Check sheet for the drawn part. Datum: minimum x, y, z corner. Units: mm. A direction names the side the tool comes from. Give positions to 0.01 mm unless a question says otherwise; leave off trailing zeros. Write each loop counter-clockwise with the first axis right and the second up, starting at its lowest first coordinate (ties: lowest second). Pieces come first, ordered by that corner, then holes. Notation, with made-up numbers: M -10,12 L -6,12 A25 ccw -6,38 Z; hole C -14,-28 d2. An arc over 180 degrees is marked long. Write item = value, one per line.
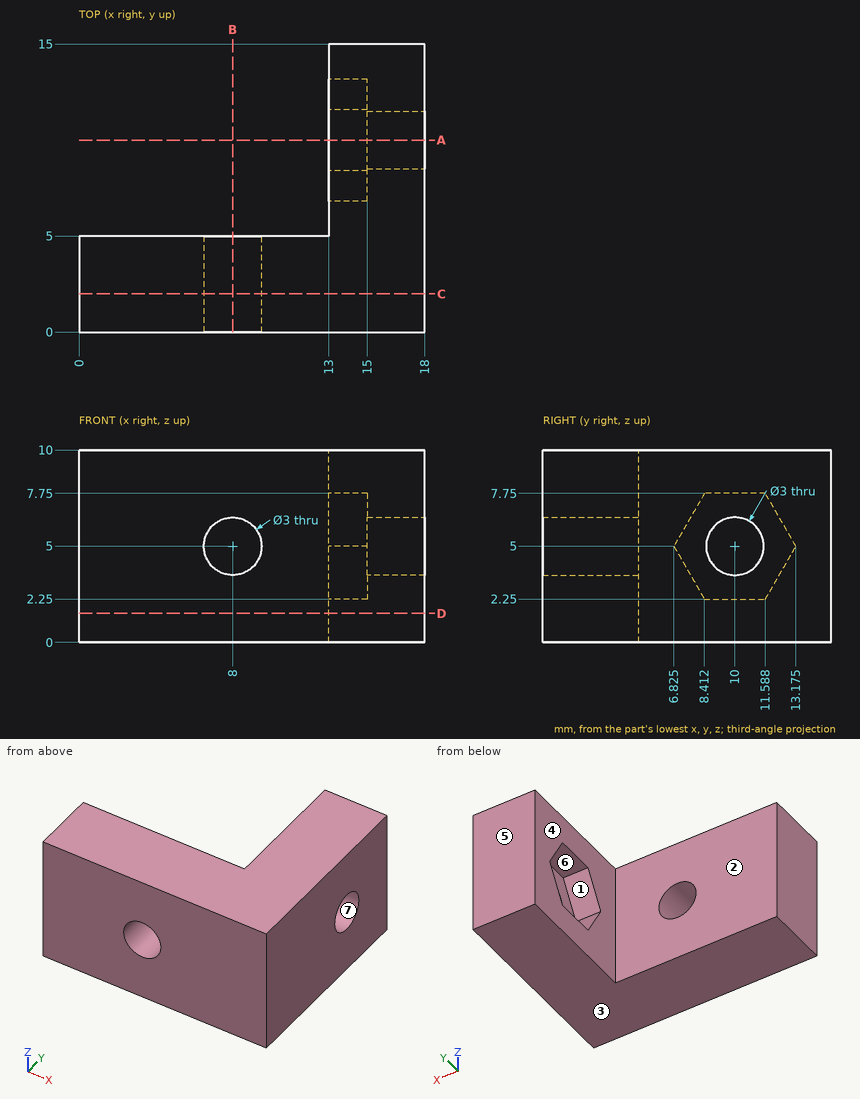
1) Cross-section at C-C on y = 2. Record the boundary of the cut face in (x, z).
From the geometry:
outline = M 0,0 L 18,0 L 18,10 L 0,10 Z; hole C 8,5 d3
2) Cross-section at A-A on y = 10. Record the boundary of the cut face in (x, z), plus the area to 3 significant figures.
From the geometry:
outline = M 13,0 L 18,0 L 18,3.5 L 15,3.5 L 15,2.25 L 13,2.25 Z; M 13,7.75 L 15,7.75 L 15,6.5 L 18,6.5 L 18,10 L 13,10 Z
area = 30.0 mm^2
3) Tool access check on the marked faces 1, 2 and 3. Record the directions out of +Z, -Z, +X, -X, +Y, -Y that give a thin tool (end or side, any length) a straight path to the whole face; none if there is none.
From the geometry:
face_1 = -X
face_2 = +Z, -Z, -X, +Y
face_3 = -Z, +X, -X, +Y, -Y
4) Material ranges on probe 1 along Y at (x, z) = (17.2, 5); probe 2 along Z at (x, y) = (8, 2.55); probe 3 along Z at (x, y) = (14, 10), recorded low to high. Write a range as from..to.
From the geometry:
probe_1 = 0..8.5, 11.5..15
probe_2 = 0..3.5, 6.5..10
probe_3 = 0..2.25, 7.75..10
5) Cross-section at D-D on z = 1.5. Record the boundary of the cut face in (x, y), plus the area to 3 significant figures.
From the geometry:
outline = M 0,0 L 18,0 L 18,15 L 13,15 L 13,5 L 0,5 Z
area = 140 mm^2
6) Draft check along Y on the marked faces 4, 5, 6 and 7. Enter one of: +Y half, -Y half, draft (parallel to the pull), parting line (faces both ways), or undercut.
From the geometry:
face_4 = draft
face_5 = +Y half
face_6 = undercut
face_7 = undercut
7) Depth check by flat-ended pin: P1, Ø5, axis at y = 9, z = 5.5, coming from the -X side; P2, Ø1.6, axis at y = 9, z = 4.5, coming from the -X side; P3, Ø5, axis at x = 4, z = 5.5, coming from the +Y side. Enter the tip coordinate at first touch or a pass-through.
From the geometry:
P1 = 13
P2 = 15
P3 = 5
8) Cross-section at B-B on x = 8. Record the boundary of the cut face in (y, z).
From the geometry:
outline = M 0,0 L 5,0 L 5,3.5 L 0,3.5 Z; M 0,6.5 L 5,6.5 L 5,10 L 0,10 Z
